```python
from build123d import *

# Parameters (mm, degrees)
ESQUISSE1_R        = 16.5
ESQUISSE1_R_2      = 11.5
BOSS_EXTRU_1_DEPTH = 4
CONG_1_R           = 3
ESQUISSE2_R        = 11
BOSS_EXTRU_2_DEPTH = 8
CONG_2_R           = 1
ESQUISSE3_R        = 13.75
BOSS_EXTRU_3_DEPTH = 36


with BuildPart() as part:
    # Esquisse1 → Boss.-Extru.1 (new body)
    with BuildSketch(Plane.XY):
        Circle(ESQUISSE1_R)
        Circle(ESQUISSE1_R_2, mode=Mode.SUBTRACT)
    extrude(amount=BOSS_EXTRU_1_DEPTH)

    # Congé1
    cong_1_edges = [part.edges().sort_by_distance(p)[0] for p in [
        (-16.5, 0, 4),
    ]]
    fillet(cong_1_edges, radius=CONG_1_R)



with BuildPart() as body_2:
    # Esquisse2 → Boss.-Extru.2 (new body)
    with BuildSketch(Plane(origin=(0, 0, 0), x_dir=(-1, 0, 0), z_dir=(0, 0, -1))):
        Circle(ESQUISSE2_R)
    extrude(amount=-BOSS_EXTRU_2_DEPTH)

    # Congé2
    cong_2_edges = [body_2.edges().sort_by_distance(p)[0] for p in [
        (11, 0, 8),
    ]]
    fillet(cong_2_edges, radius=CONG_2_R)


with BuildPart() as part_1:
    add(part.part)

    add(body_2.part)  # Boss.-Extru.3 merges body 2
    # Esquisse3 → Boss.-Extru.3 (add)
    with BuildSketch(Plane(origin=(0, 0, 0), x_dir=(-1, 0, 0), z_dir=(0, 0, -1))):
        with Locations(Location((0, 0, 0), (0, 0, 180))):
            Circle(ESQUISSE3_R)
    extrude(amount=BOSS_EXTRU_3_DEPTH)


solid = part_1.part
```
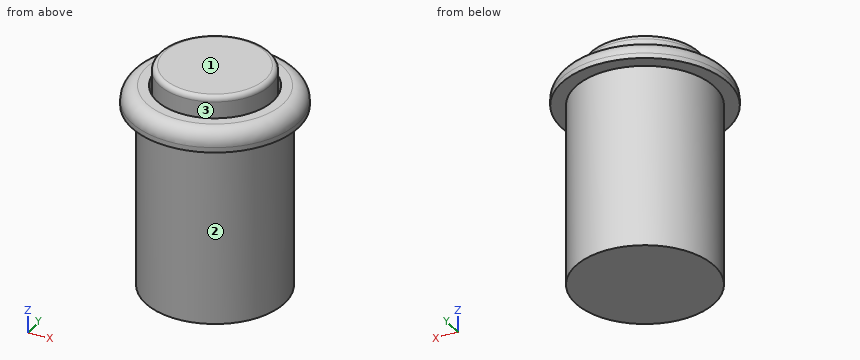
Check sheet for the modelled part. Datum: model origin and axes. Units: mm. Face numbers are marked on the shaded views. Coordinates: 2 decimals unless noted, no trailing zeros. Write each loop counter-clockwise with the first axis right and the second up, starting at its lowest first coordinate (ties: lowest second). Pieces come first, ordered by that corner, then holes. Notation, with made-up numbers: M 43.25,1 L 94.25,1 A30 ccw 94.25,32 Z; hole C 32,-40 d9. An arc over 180 degrees is marked long. Write item = value, one per line. Start each with the question number.
1. Sectioned sample at A-A (y = 0). Record the cut outline in (x, z), then the cut area to 3 significant figures.
2. Go/stop test with flat-tipped pins: pin 1 (6 mm diameter, centred on x = 6.5, y = -13, fed in from +Z); pin 2 (4 mm diameter, centred on y = -11, z = -7.5, fed in from -X); pin 3 (4 mm diameter, centred on y = 2, z = -10, fed in from +X). Record where each tip stops, or that it passes through.
3. Sectioned sample at C-C (z = -12). Record the cut outline in (x, y).
4. Mould release check, pull along X, two halves, no side actions. Record for the marked faces 1, 2 and 3: pulls with the +X half, pulls with the -X half, needs draft (parallel to the pull), parting line crosses it, or undercut.
5. Thickness scan on probe 1 along Y at (x, z) = (0, 1); probe 2 along Y at (x, z) = (0, 2.3); probe 3 along Z at (x, y) = (-4.5, -11). Record the ranges inside material, lowest first.
The answers:
q1.outline = M -16.5,0 L -13.75,0 L -13.75,-36 L 13.75,-36 L 13.75,0 L 16.5,0 L 16.5,1 A3 ccw 13.5,4 L 11.5,4 L 11.5,0 L 11,0 L 11,7 A1 ccw 10,8 L -10,8 A1 ccw -11,7 L -11,0 L -11.5,0 L -11.5,4 L -13.5,4 A3 ccw -16.5,1 Z
q1.area = 1,200 mm²
q2.pin_1 = 4
q2.pin_2 = -10.4
q2.pin_3 = 13.75
q3.outline = C 0,0 d27.5
q4.face_1 = needs draft
q4.face_2 = parting line crosses it
q4.face_3 = undercut
q5.probe_1 = -16.5 to -11.5, -11 to 11, 11.5 to 16.5
q5.probe_2 = -16.2 to -11.5, -11 to 11, 11.5 to 16.2
q5.probe_3 = -36 to 4
